Source: three-view drawing plus pictorial views. Frame: mm from the lowest corner of the part. Give positions to 0.01 mm unless a question says otherwise; leave off trailing zeros. Order: outer loops, then holes, each group sorted by start corner. A loop starts at its lowest first (then second) coordinate and runs counter-clockwise, first axis right, second up. Notation, with made-up numbers: (80.5, 54) - (111.5, 54) arc R32 cw to (111.5, 91) - close; hole circle Ø11 at (6, -15.5). An arc over 180 degrees is marked (long way). Answer in a Markdown table with one row per item. Add a question column.
1. Contact query for flat-ended pins moving along their axis: pin 1 (1.2 mm diameter, centred on x = 29, y = 25.5, fed in from -Z); pin 2 (2 mm diameter, centred on x = 29.5, y = 14, fed in from -Z). Output: stop coordinate, or through.
2. Section query C-C on x = 17. Return loops of the section in (y, z).
3. Section query B-B on z = 15. Return loops of the section in (x, y).
4. Mould query, pull axis X, two halves, no side actions, for the marked faces 1, 2 and 3. Classes: released by +X, released by -X, zero draft, split by the parting line, or undercut.
5. Section query D-D on x = 29.25. Return loops of the section in (y, z).
6. Section query A-A on y = 4.75. Return loops of the section in (x, z), and give its area (3 significant figures).
7. Ray query, line 1 (X direction, y = 4.75, z = 5.75); line 2 (Y direction, x = 29.25, z = 4); line 3 (X direction, y = 16.25, z = 15). Return the intervals inside material, ascending. Write a range as [from, to].
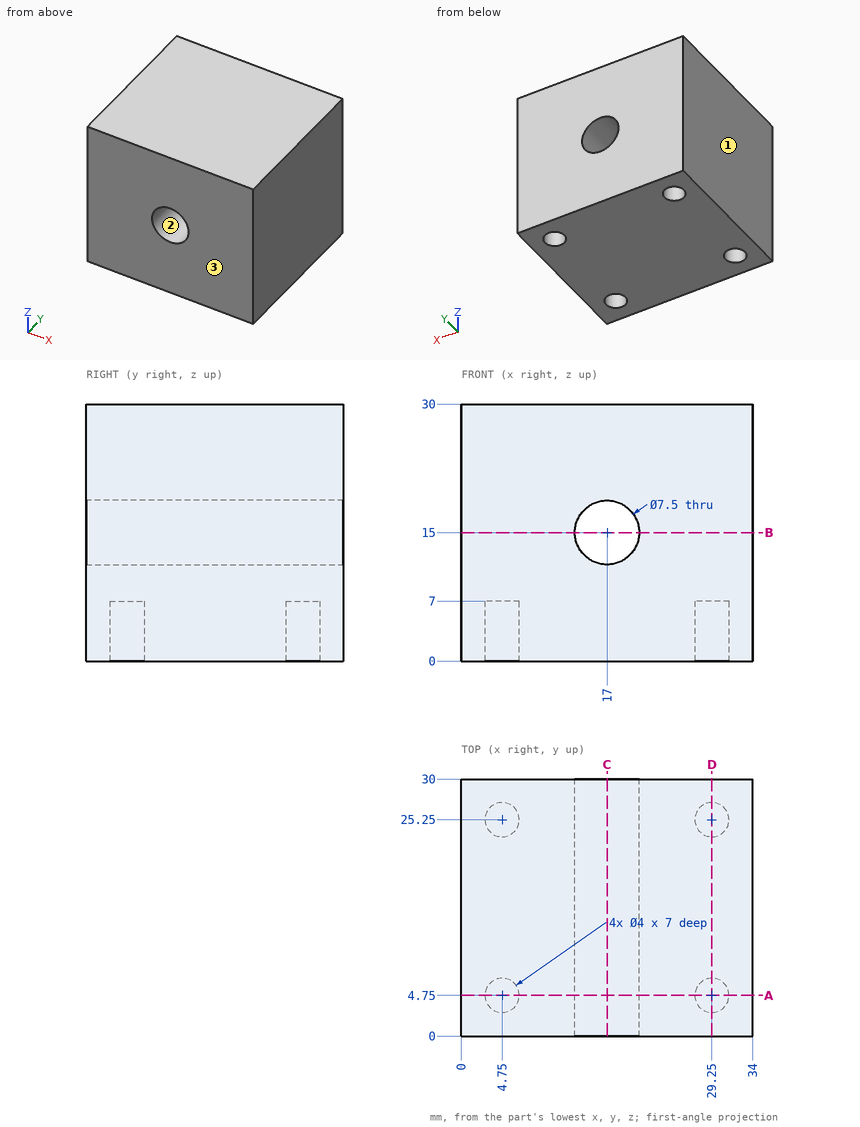
Answer:
| question | item | result |
|---|---|---|
| 1 | pin 1 | stops at z = 7 |
| 1 | pin 2 | stops at z = 0 |
| 2 | outline | (0, 0) - (30, 0) - (30, 11.25) - (0, 11.25) - close; (0, 18.75) - (30, 18.75) - (30, 30) - (0, 30) - close |
| 3 | outline | (0, 0) - (13.25, 0) - (13.25, 30) - (0, 30) - close; (20.75, 0) - (34, 0) - (34, 30) - (20.75, 30) - close |
| 4 | face 1 | released by -X |
| 4 | face 2 | undercut |
| 4 | face 3 | zero draft |
| 5 | outline | (0, 0) - (2.75, 0) - (2.75, 7) - (6.75, 7) - (6.75, 0) - (23.25, 0) - (23.25, 7) - (27.25, 7) - (27.25, 0) - (30, 0) - (30, 30) - (0, 30) - close |
| 6 | outline | (0, 0) - (2.75, 0) - (2.75, 7) - (6.75, 7) - (6.75, 0) - (27.25, 0) - (27.25, 7) - (31.25, 7) - (31.25, 0) - (34, 0) - (34, 30) - (0, 30) - close; hole circle Ø7.5 at (17, 15) |
| 6 | area | 920 mm² |
| 7 | line 1 | x = [0, 2.75], [6.75, 27.25], [31.25, 34] |
| 7 | line 2 | y = [0, 2.75], [6.75, 23.25], [27.25, 30] |
| 7 | line 3 | x = [0, 13.25], [20.75, 34] |
